Model file for the job. Use its own axes, mm. Face numbers are marked on the shaded views. A direction names the side the tool comes from. Coordinates: 2 decimals unless noted, no trailing zeros.
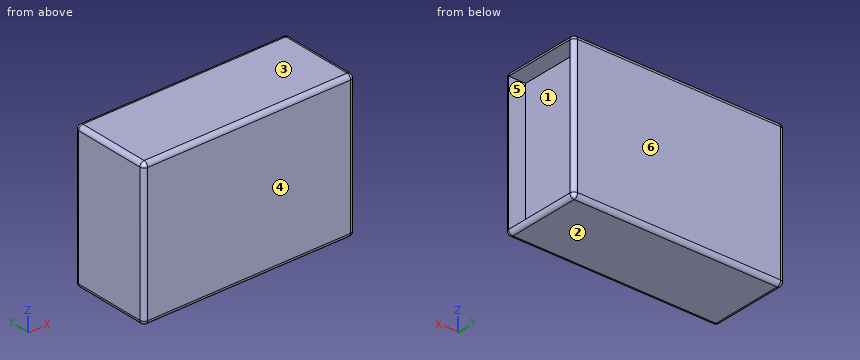
from build123d import *

# Parameters (mm, degrees)
SKETCH1_W           = 50
SKETCH1_H           = 34
BOSS_EXTRUDE1_DEPTH = 19
SKETCH2_W           = 32
SKETCH2_H           = 17
CUT_EXTRUDE1_DEPTH  = 4
FILLET1_R           = 1
FILLET2_R           = 1


# Some blends are built 0.0001 mm under size
with BuildPart() as part:
    # Sketch1 → Boss-Extrude1 (new body)
    with BuildSketch(Plane(origin=(0, 0, 0), x_dir=(1, 0, 0), z_dir=(0, 1, 0))):
        Rectangle(SKETCH1_W, SKETCH1_H)
    extrude(amount=BOSS_EXTRUDE1_DEPTH)

    # Sketch2 → Cut-Extrude1 (cut)
    with BuildSketch(Plane(origin=(25, 0, 0), x_dir=(0, 0, -1), z_dir=(1, 0, 0))):
        with Locations((0, 9.5)):
            Rectangle(SKETCH2_W, SKETCH2_H)
    extrude(amount=-CUT_EXTRUDE1_DEPTH, mode=Mode.SUBTRACT)

    # Fillet1
    fillet1_edges = [part.edges().sort_by_distance(p)[0] for p in [
        (-25, 19, 0),
        (0, 19, 17),
        (25, 19, 0),
        (0, 0, 17),
        (-25, 0, 0),
        (0, 0, -17),
        (25, 0, 0),
        (0, 19, -17),
        (25, 9.5, 17),
        (25, 9.5, -17),
    ]]
    fillet(fillet1_edges, radius=FILLET1_R - 0.0001)  # a hair under: the kernel refuses the full size

    # Fillet2
    # the kernel refuses this fillet: 1 mm, written as the material it takes off along each edge
    with BuildSketch(Plane(origin=(-24, 19, -16), x_dir=(0, 0, -1), z_dir=(1, 0, 0))) as fillet2_piece_1:
        with BuildLine():
            CenterArc((0.0001, -0.9999), 0.9999, 0, 90)
            Line((1, -0.9999), (1, 0))
            Line((1, 0), (0.0001, 0))
        make_face()
    revolve(axis=Axis((-24, 19, -16), (0, 1, 0)), revolution_arc=90, mode=Mode.SUBTRACT)
    with BuildSketch(Plane(origin=(-24, 19, 16), x_dir=(-1, 0, 0), z_dir=(0, 0, -1))) as fillet2_piece_2:
        with BuildLine():
            CenterArc((0.0001, -0.9999), 0.9999, 0, 90)
            Line((1, -0.9999), (1, 0))
            Line((1, 0), (0.0001, 0))
        make_face()
    revolve(axis=Axis((-24, 19, 16), (0, 1, 0)), revolution_arc=90, mode=Mode.SUBTRACT)
    with BuildSketch(Plane(origin=(-24, 0, -16), x_dir=(-1, 0, 0), z_dir=(0, 0, 1))) as fillet2_piece_3:
        with BuildLine():
            CenterArc((0.0001, -0.9999), 0.9999, 0, 90)
            Line((1, -0.9999), (1, 0))
            Line((1, 0), (0.0001, 0))
        make_face()
    revolve(axis=Axis((-24, 0, -16), (0, -1, 0)), revolution_arc=90, mode=Mode.SUBTRACT)
    with BuildSketch(Plane(origin=(-24, 0, 16), x_dir=(0, 0, 1), z_dir=(1, 0, 0))) as fillet2_piece_4:
        with BuildLine():
            CenterArc((0.0001, -0.9999), 0.9999, 0, 90)
            Line((1, -0.9999), (1, 0))
            Line((1, 0), (0.0001, 0))
        make_face()
    revolve(axis=Axis((-24, 0, 16), (0, -1, 0)), revolution_arc=90, mode=Mode.SUBTRACT)
    with BuildSketch(Plane(origin=(-25, 0, 17), x_dir=(0, 0, -1), z_dir=(0, 1, 0)), Plane(origin=(-25, 0, -17), x_dir=(1, 0, 0), z_dir=(0, 1, 0))) as fillet2_piece_5:
        with BuildLine():
            CenterArc((FILLET2_R, -FILLET2_R), FILLET2_R, 90, 90)
            Line((0, -FILLET2_R), (0, 0))
            Line((0, 0), (FILLET2_R, 0))
        make_face()
    extrude(amount=19, mode=Mode.SUBTRACT)


solid = part.part
Q1. Mould opens along Z. For the marked faces 1, 2, 3 and 4 say: +Z half, -Z half, draft (parallel to the pull), parting line (faces both ways), or undercut.
Answers:
face 1: undercut
face 2: -Z half
face 3: +Z half
face 4: draft
Q2. Which spindle directions (+Z, -Z, +X, -X, +Y, -Y) get a long thin tool onto all of the face, cutting with end or side? Do the marked faces 5 and 6. Say none if no direction does.
Answers:
face 5: +X
face 6: +Z, -Z, +X, -X, +Y
Q3. Drill centre lines: line 1 (Y direction, x = 22.5, z = -1); line 2 (X direction, y = 5, z = -14). Where is each one in solid material? Low to high.
Answers:
line 1: y = 0 to 1, 18 to 19
line 2: x = -25 to 21
Q4. Flat gauge pins, fed straight in: P1, Ø6, axis at y = 13, z = 6.5, coming from the +X side; P2, Ø8, axis at y = 2.5, z = 8, coming from the +X side. Where does each tip first touch, or does it go through?
Answers:
P1: stops at x = 21
P2: stops at x = 25
